Geometry: final body of the model. Coordinates: model frame, mm. A direction names the side the tool comes from. Give positions to 0.01 mm unless a question says otherwise; leave off trailing zeros. Write each loop counter-clockwise with the first axis right and the second up, starting at its lowest first coordinate (ties: lowest second). Pieces come first, ordered by that corner, then holes.
Q1. Section C-C (y = -3). Return the cut outline in (x, z).
Q2. Mould query, pull axis Y, two halves, no side actions, for faces 3 (the cylindrical face through (-3.37, -4.75, 0.08)), 4 (the flat face through (0, 0, 0)), 5 (the flat face through (0, 3, 0)). Classes: +Y half, -Y half, draft (parallel to the pull), parting line (faces both ways), or undercut.
Q3. Reachability of faces 1 (the flat face through (2, -7, -2)), 2 (the cylindrical face through (-0.54, -3.45, -2.44)) from +Z, -Z, +X, -X, +Y, -Y: full face, straight path, thin tool, end or side. Return the list, or none.
Q4. Pin query (flat end, axial travel): pin 1 Ø5.5 at (y, z) = (-3, 0) entering from -X; pin 2 Ø1.5 at (y, z) = (0.5, 3.5) entering from -X; pin 3 Ø2 at (y, z) = (-3, 0) entering from +X; pin 4 Ø3 at (y, z) = (-4, 2) entering from +X. Return the tip coordinate at first contact, or that it passes through.
Q5. Section B-B (x = 0). Return the cut outline in (y, z).
Q6. Line query: line 1 (Z direction, x = 0, y = -2); line 2 (Y direction, x = 4.15, z = 0); line 3 (Z direction, x = -1.25, y = -1). Output: solid intervals per line, ascending.
Q7. Section A-A (z = 0). Return the cut outline in (x, y), plus the area to 3 significant figures.
Q8. Section D-D (x = 3). Return the cut outline in (y, z).
from build123d import *

# Parameters (mm, degrees)
F0_R     = 5
F0_R_2   = 2.5
F1_DEPTH = 7
F2_R     = 5
F3_DEPTH = 3
F4_R     = 1.75
F5_DEPTH = 12.5


with BuildPart() as f1:
    # F0 (on Front) → F1 (new body)
    with BuildSketch(Plane.XZ):
        Circle(F0_R)
        Circle(F0_R_2, mode=Mode.SUBTRACT)
    extrude(amount=F1_DEPTH)

    # F2 (on Front) → F3 (join)
    with BuildSketch(Plane.XZ):
        Circle(F2_R)
    extrude(amount=-F3_DEPTH)

    # F4 (on Right) → F5 (cut, symmetric)
    with BuildSketch(Plane.YZ):
        with Locations((-3, 0)):
            Circle(F4_R)
    extrude(amount=F5_DEPTH, both=True, mode=Mode.SUBTRACT)


solid = f1.part
Computed:
1. outline: (-4.68, -1.75) arc R5 ccw to (4.68, -1.75) - (1.79, -1.75) arc R2.5 cw to (-1.79, -1.75) - close; (-4.68, 1.75) - (-1.79, 1.75) arc R2.5 cw to (1.79, 1.75) - (4.68, 1.75) arc R5 ccw to start
2. face 3: undercut
2. face 4: -Y half
2. face 5: +Y half
3. face 1: +Z, -Z, +X, -X, -Y
3. face 2: -Y
4. pin 1: stops at x = -5
4. pin 2: stops at x = -4.18
4. pin 3: passes through
4. pin 4: stops at x = 4.96
5. outline: (-7, -5) - (3, -5) - (3, 5) - (-7, 5) - (-7, 2.5) - (0, 2.5) - (0, -2.5) - (-7, -2.5) - close
6. line 1: z = -5 to -2.5, 2.5 to 5
6. line 2: y = -7 to -4.75, -1.25 to 3
6. line 3: z = -4.84 to -2.17, 2.17 to 4.84
7. outline: (-5, -7) - (-2.5, -7) - (-2.5, -4.75) - (-5, -4.75) - close; (-5, -1.25) - (-2.5, -1.25) - (-2.5, 0) - (2.5, 0) - (2.5, -1.25) - (5, -1.25) - (5, 3) - (-5, 3) - close; (2.5, -7) - (5, -7) - (5, -4.75) - (2.5, -4.75) - close
7. area: 47.5 mm2
8. outline: (-7, -4) - (3, -4) - (3, 4) - (-7, 4) - close; hole circle Ø3.5 at (-3, 0)
